from build123d import *

# Parameters (mm, degrees)
SKETCH1_W           = 183
SKETCH1_H           = 118
SKETCH1_W_2         = 21
SKETCH1_H_2         = 41.5
BOSS_EXTRUDE1_DEPTH = 5
SKETCH2_R           = 0.75
SKETCH2_R_2         = 0.865315656
CUT_EXTRUDE1_DEPTH  = 5
FILLET5_R           = 10
FILLET6_R           = 10
FILLET7_R           = 10
FILLET8_R           = 10


with BuildPart() as part:
    # Sketch1 → Boss-Extrude1 (new body)
    with BuildSketch(Plane.XY):
        with Locations((-91.5, 59)):
            Rectangle(SKETCH1_W, SKETCH1_H)
        with Locations((-162.5, 28.25)):
            Rectangle(SKETCH1_W_2, SKETCH1_H_2, mode=Mode.SUBTRACT)
        with Locations((-91.5, 28.25)):
            Rectangle(SKETCH1_W_2, SKETCH1_H_2, mode=Mode.SUBTRACT)
        with Locations((-20.5, 28.25)):
            Rectangle(SKETCH1_W_2, SKETCH1_H_2, mode=Mode.SUBTRACT)
        with Locations((-162.5, 89.75)):
            Rectangle(SKETCH1_W_2, SKETCH1_H_2, mode=Mode.SUBTRACT)
        with Locations((-91.5, 89.75)):
            Rectangle(SKETCH1_W_2, SKETCH1_H_2, mode=Mode.SUBTRACT)
        with Locations((-20.5, 89.75)):
            Rectangle(SKETCH1_W_2, SKETCH1_H_2, mode=Mode.SUBTRACT)
    extrude(amount=BOSS_EXTRUDE1_DEPTH)

    # Sketch2 → Cut-Extrude1 (cut)
    with BuildSketch(Plane.XY.offset(5)):
        with Locations((-167.5, 114.9)):
            Circle(SKETCH2_R)
        with Locations((-157.5, 114.9)):
            Circle(SKETCH2_R_2)
        with Locations((-167.5, 64.6)):
            Circle(SKETCH2_R)
        with Locations((-157.5, 64.6)):
            Circle(SKETCH2_R)
        with Locations((-96.5, 114.9)):
            Circle(SKETCH2_R)
        with Locations((-86.5, 114.9)):
            Circle(SKETCH2_R_2)
        with Locations((-96.5, 64.6)):
            Circle(SKETCH2_R)
        with Locations((-86.5, 64.6)):
            Circle(SKETCH2_R_2)
        with Locations((-96.5, 53.4)):
            Circle(SKETCH2_R)
        with Locations((-86.5, 53.4)):
            Circle(SKETCH2_R_2)
        with Locations((-25.5, 114.9)):
            Circle(SKETCH2_R)
        with Locations((-15.5, 114.9)):
            Circle(SKETCH2_R_2)
        with Locations((-25.5, 64.6)):
            Circle(SKETCH2_R)
        with Locations((-15.5, 64.6)):
            Circle(SKETCH2_R_2)
        with Locations((-25.5, 53.4)):
            Circle(SKETCH2_R)
        with Locations((-15.5, 53.4)):
            Circle(SKETCH2_R_2)
        with Locations((-25.5, 3.1)):
            Circle(SKETCH2_R)
        with Locations((-15.5, 3.1)):
            Circle(SKETCH2_R_2)
        with Locations((-96.5, 3.1)):
            Circle(SKETCH2_R)
        with Locations((-86.5, 3.1)):
            Circle(SKETCH2_R_2)
        with Locations((-167.5, 3.1)):
            Circle(SKETCH2_R)
        with Locations((-157.5, 3.1)):
            Circle(SKETCH2_R_2)
        with Locations((-167.5, 53.4)):
            Circle(SKETCH2_R)
        with Locations((-157.5, 53.4)):
            Circle(SKETCH2_R_2)
    extrude(amount=-CUT_EXTRUDE1_DEPTH, mode=Mode.SUBTRACT)

    # Fillet5
    fillet5_edges = [part.edges().sort_by_distance(p)[0] for p in [
        (-183, 118, 2.5),
    ]]
    fillet(fillet5_edges, radius=FILLET5_R)

    # Fillet6
    fillet6_edges = [part.edges().sort_by_distance(p)[0] for p in [
        (-183, 0, 2.5),
    ]]
    fillet(fillet6_edges, radius=FILLET6_R)

    # Fillet7
    fillet7_edges = [part.edges().sort_by_distance(p)[0] for p in [
        (0, 118, 2.5),
    ]]
    fillet(fillet7_edges, radius=FILLET7_R)

    # Fillet8
    fillet8_edges = [part.edges().sort_by_distance(p)[0] for p in [
        (0, 0, 2.5),
    ]]
    fillet(fillet8_edges, radius=FILLET8_R)


solid = part.part
Model file for the job. Use its own axes, mm. A direction names the side the tool comes from. Give positions to 0.01 mm unless a question says otherwise; leave off trailing zeros. Order: outer loops, then holes, each group sorted by start corner. A loop starts at its lowest first (then second) coordinate and runs counter-clockwise, first axis right, second up. Notation, with made-up numbers: (-34.5, -13.5) -> (12.5, -13.5) arc R29 cw to (12.5, 8.5) -> close; hole circle Ø10 at (24, 80.25). An arc over 180 degrees is marked (long way). Use CSV: the item, a comma, the result in double quotes.
1. Drill centre lines: line 1 along Y through (x, z) = (-172, 2); line 2 along X through (y, z) = (77.5, 1.3); line 3 along X through (y, z) = (5, 2.9). Where is each one in solid material? Low to high. Write a range as from..to.
Outcome:
line 1,"0..7.5, 49..69, 110.5..118"
line 2,"-183..-173, -152..-102, -81..-31, -10..0"
line 3,"-181.66..-1.34"
2. Band-saw the part on B-B, the plane z = 2.6. Count the separate pieces of the cut face and the enclosed holes in it, then the cut area to 3 significant figures.
Outcome:
separate pieces,"1"
enclosed holes,"30"
area,"16,200 mm²"
3. Mould opens along Y. For faces 1 (the flat face through (-93, 0, 2)), 2 (the flat face through (-93, 60, 0)), 3 (the flat face through (-92, 110.5, 2)) say: +Y half, -Y half, draft (parallel to the pull), parting line (faces both ways), or undercut.
Outcome:
face 1,"-Y half"
face 2,"draft"
face 3,"undercut"
4. Band-saw the part on A-A, the plane y = 13. Give the cut face in (x, z).
Outcome:
outline,"(-183, 0) -> (-173, 0) -> (-173, 5) -> (-183, 5) -> close; (-152, 0) -> (-102, 0) -> (-102, 5) -> (-152, 5) -> close; (-81, 0) -> (-31, 0) -> (-31, 5) -> (-81, 5) -> close; (-10, 0) -> (0, 0) -> (0, 5) -> (-10, 5) -> close"
5. 3-axis set-ups, long thin cutter, end or side, ignore diameter. For faces 4 (the flat face through (-93, 60, 5)), 5 (the flat face through (-102, 89, 2)): which of +Z, -Z, +X, -X, +Y, -Y reach the whole face in a straight line?
Outcome:
face 4,"+Z, +X, -X, +Y, -Y"
face 5,"+Z, -Z"
